Verification items for this drawing (mm, ordinates from the low corner). A direction names the side the tool comes from. Coordinates: 2 decimals unless noted, no trailing zeros. Order: outer loops, then holes, each group sorted by start corner. A loop starts at its lowest first (then second) coordinate and runs counter-clockwise, first axis right, second up.
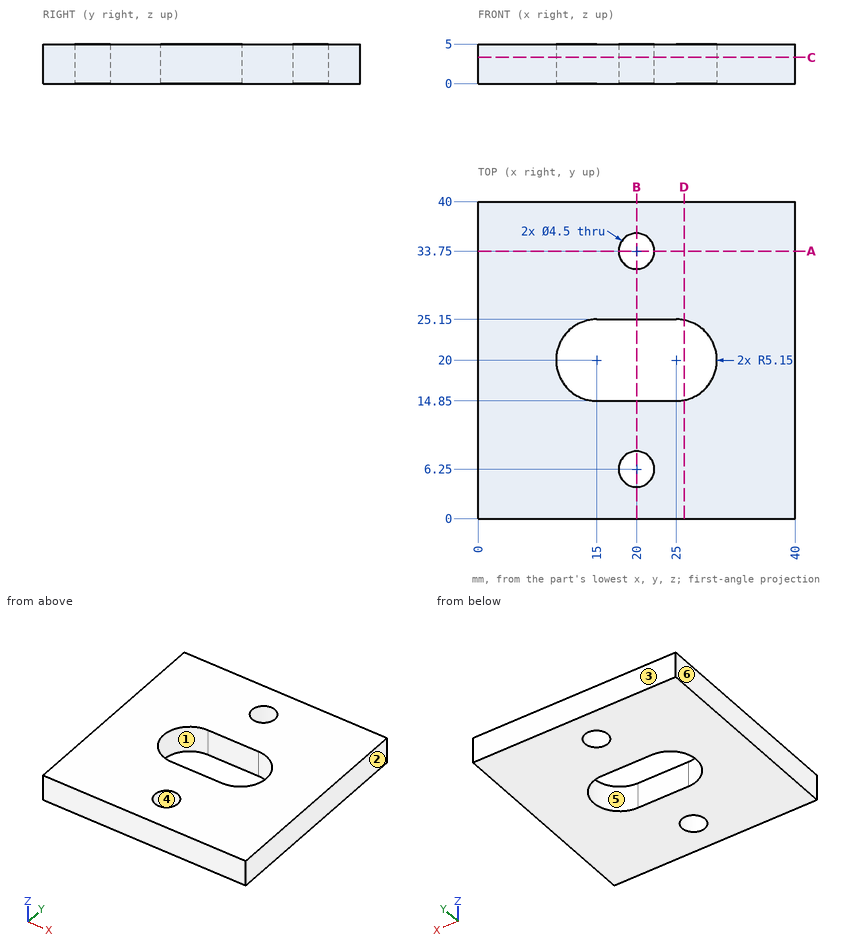
Item 1: Thickness scan on line 1 along Y through (x, z) = (20, 1.45); line 2 along X through (y, z) = (32.5, 4.1); line 3 along Y through (x, z) = (14, 2.15). Record the ranges inside material, lowest first.
Item 2: Sectioned sample at C-C (z = 3.3). Record the cut outline in (x, y).
Item 3: Release check for a two-part mould opening along Y. For the marked faces 1, 2, 3 and 4 record: pulls with the +Y half, pulls with the -Y half, needs draft (parallel to the pull), parting line crosses it, or undercut.
Item 4: Depth check by flat-ended pin: P1, Ø2.5, axis at x = 20, z = 1.5, coming from the -Y side. Enter the tip coordinate at first touch or a pass-through.
Item 5: Sectioned sample at B-B (x = 20). Record the cut outline in (y, z).
Item 6: Sectioned sample at D-D (x = 26). Record the cut outline in (y, z), and give its area (3 significant figures).
Item 7: Sectioned sample at A-A (y = 33.75). Record the cut outline in (x, z).
Item 8: Tool access check on the marked faces 5 and 6. Record the directions out of +Z, -Z, +X, -X, +Y, -Y that give a thin tool (end or side, any length) a straight path to the whole face; none if there is none.
Geometry check:
1. line 1: y = 0 to 4, 8.5 to 14.85, 25.15 to 31.5, 36 to 40
1. line 2: x = 0 to 18.13, 21.87 to 40
1. line 3: y = 0 to 14.95, 25.05 to 40
2. outline: (0, 0) - (40, 0) - (40, 40) - (0, 40) - close; hole (15, 14.85) - (25, 14.85) arc R5.15 ccw to (25, 25.15) - (15, 25.15) arc R5.15 ccw to start; hole circle Ø4.5 at (20, 6.25); hole circle Ø4.5 at (20, 33.75)
3. face 1: undercut
3. face 2: needs draft
3. face 3: pulls with the +Y half
3. face 4: undercut
4. P1: stops at y = 0
5. outline: (0, 0) - (4, 0) - (4, 5) - (0, 5) - close; (8.5, 0) - (14.85, 0) - (14.85, 5) - (8.5, 5) - close; (25.15, 0) - (31.5, 0) - (31.5, 5) - (25.15, 5) - close; (36, 0) - (40, 0) - (40, 5) - (36, 5) - close
6. outline: (0, 0) - (14.95, 0) - (14.95, 5) - (0, 5) - close; (25.05, 0) - (40, 0) - (40, 5) - (25.05, 5) - close
6. area: 149 mm2
7. outline: (0, 0) - (17.75, 0) - (17.75, 5) - (0, 5) - close; (22.25, 0) - (40, 0) - (40, 5) - (22.25, 5) - close
8. face 5: +Z, -Z
8. face 6: +Z, -Z, -X, +Y, -Y
